Could you check a few things on this model? Use its own coordinates, in mm. A direction names the side the tool comes from. Coordinates: 2 decimals unless noted, no trailing zeros. Order: outer loops, then holes, each group sorted by start corner. A loop starts at its lowest first (then second) coordinate and runs counter-clockwise, first axis right, second up. Notation, with made-up numbers: (-5, 76) -> (10, 76) arc R13 ccw to (10, 88) -> close; hole circle Ø3 at (60, 3). An arc over 180 degrees is marked (long way). Use a Markdown table: item, result. Add a question column.
1) If we section it at C-C (x = -18): Write out the boundary of the cut face in (y, z).
2) Will these pins go through, and if not, where does the flat tip stop? pin 1 Ø0.8 at (y, z) = (5.5, 0.5) entering from +X; pin 2 Ø0.5 at (y, z) = (4.5, 0.5) entering from -X; pin 3 Ø0.5 at (x, z) = (-13.5, 1) entering from +Y; pin 4 Ø2.5 at (x, y) = (0, 18.415) entering from +Z.
3) If we section it at D-D (z = 0.9): Write out the boundary of the cut face in (x, y) (1 decimal), plus the area to 3 significant figures.
4) If we section it at A-A (x = 0): Write out the boundary of the cut face in (y, z), plus the area to 3 significant figures.
5) Which directions (+Z, -Z, +X, -X, +Y, -Y) give clear straight access to the entire face, cutting with the end or side of a thin tool? Please do faces 5 (the flat face through (-16.984, -4, 1)), 6 (the flat face through (0, -4, 0)), 7 (the flat face through (-2.007, -10.091, 0.783)).
6) Thinking about a two-plate mould opening in X: for faces 1 (the flat face through (-19, -5.524, 1)), 2 (the flat face through (-7.925, 5, 1)), 3 (the cylindrical face through (21.572, -0.871, 0.783)), 4 (the flat face through (-16.984, 4, 1)), which applies, +X half, -X half, draft (parallel to the pull), parting line (faces both ways), or undercut?
7) If I drill on L1, parallel to Y at x = 0, z = 1.05; L2, parallel to X at y = 6, z = 1.35; L3, parallel to X at y = 0, z = 1, over which ranges is the centre line in solid material (lowest first)? Write a range as [from, to].
8) If we section it at B-B (y = 0): Write out the boundary of the cut face in (x, z).
```python
from build123d import *

# Parameters (mm, degrees)
SKETCH1_R           = 1.4224
BOSS_EXTRUDE2_DEPTH = 1.5875


with BuildPart() as part:
    # Sketch1 → Boss-Extrude2 (new body)
    with BuildSketch(Plane.XY):
        with BuildLine():
            Line((-7.9248, 3.302), (-11.65986156, 2.948480848))
            Line((-11.65986156, 2.948480848), (-11.65986156, -2.948480848))
            Line((-11.65986156, -2.948480848), (-16.984058744, -2.948480848))
            Line((-16.984058744, -2.948480848), (-16.984058744, -5.5245))
            Line((-16.984058744, -5.5245), (-20.871224203, -5.5245))
            ThreePointArc((-20.871224203, -5.5245), (21.59, 0), (-20.871224203, 5.5245))
            Line((-20.871224203, 5.5245), (-16.984058744, 5.5245))
            Line((-16.984058744, 5.5245), (-16.984058744, 2.948480848))
            Line((-16.984058744, 2.948480848), (-14.952058744, 2.948480848))
            ThreePointArc((-14.952058744, 2.948480848), (-13.968818521, 6.093415226), (-12.332576282, 8.9535))
            Line((-12.332576282, 8.9535), (-7.9248, 7.366))
            Line((-7.9248, 7.366), (-7.9248, 3.302))
        make_face()
        with Locations((0, -18.415)):
            Circle(SKETCH1_R, mode=Mode.SUBTRACT)
        Polygon((-10.36446156, -3.837480848), (-8.512343898, -1.936173756), (-2.917588579, -7.386185056), (-2.594132624, -7.054138602), (-0.7747, -8.8265), (-3.273729572, -11.3919), (-5.093162196, -9.619538602), (-4.769706241, -9.287492148), align=None, mode=Mode.SUBTRACT)
        with Locations((0, 18.415)):
            Circle(SKETCH1_R, mode=Mode.SUBTRACT)
        with BuildLine():
            Line((11.43, 14.6558), (11.43, -0.8128))
            Line((11.43, -0.8128), (-5.6007, -0.8128))
            Line((-5.6007, -0.8128), (-5.6007, 14.173558463))
            ThreePointArc((-5.6007, 14.173558463), (-4.895856129, 14.43219293), (-4.179129857, 14.6558))
            Line((-4.179129857, 14.6558), (4.179129857, 14.6558))
            Line((4.179129857, 14.6558), (11.43, 14.6558))
        make_face(mode=Mode.SUBTRACT)
    extrude(amount=BOSS_EXTRUDE2_DEPTH)


solid = part.part
```
Answer sheet:
| question | item | result |
|---|---|---|
| 1 | outline | (-11.92, 0) -> (-5.52, 0) -> (-5.52, 1.59) -> (-11.92, 1.59) -> close; (5.52, 0) -> (11.92, 0) -> (11.92, 1.59) -> (5.52, 1.59) -> close |
| 2 | pin 1 | x = 20.98 |
| 2 | pin 2 | x = -16.98 |
| 2 | pin 3 | y = 17.05 |
| 2 | pin 4 | through |
| 3 | outline | (-20.9, -5.5) arc R21.6 ccw (long way) to (-20.9, 5.5) -> (-17, 5.5) -> (-17, 2.9) -> (-15, 2.9) arc R15.2 cw to (-12.3, 9) -> (-7.9, 7.4) -> (-7.9, 3.3) -> (-11.7, 2.9) -> (-11.7, -2.9) -> (-17, -2.9) -> (-17, -5.5) -> close; hole (-10.4, -3.8) -> (-4.8, -9.3) -> (-5.1, -9.6) -> (-3.3, -11.4) -> (-0.8, -8.8) -> (-2.6, -7.1) -> (-2.9, -7.4) -> (-8.5, -1.9) -> close; hole (-5.6, -0.8) -> (11.4, -0.8) -> (11.4, 14.7) -> (-4.2, 14.7) arc R15.2 ccw to (-5.6, 14.2) -> close; hole circle Ø2.8 at (0, -18.4); hole circle Ø2.8 at (0, 18.4) |
| 3 | area | 1,050 mm2 |
| 4 | outline | (-21.59, 0) -> (-19.84, 0) -> (-19.84, 1.59) -> (-21.59, 1.59) -> close; (-16.99, 0) -> (-0.81, 0) -> (-0.81, 1.59) -> (-16.99, 1.59) -> close; (14.66, 0) -> (16.99, 0) -> (16.99, 1.59) -> (14.66, 1.59) -> close; (19.84, 0) -> (21.59, 0) -> (21.59, 1.59) -> (19.84, 1.59) -> close |
| 4 | area | 35.0 mm2 |
| 5 | face 5 | +Z, -Z, -X |
| 5 | face 6 | -Z, +X, -X, +Y, -Y |
| 5 | face 7 | +Z, -Z |
| 6 | face 1 | draft |
| 6 | face 2 | undercut |
| 6 | face 3 | parting line |
| 6 | face 4 | -X half |
| 7 | L1 | [-21.59, -19.84], [-16.99, -0.81], [14.66, 16.99], [19.84, 21.59] |
| 7 | L2 | [-20.74, -14.01], [-7.92, -5.6], [11.43, 20.74] |
| 7 | L3 | [-11.66, -5.6], [11.43, 21.59] |
| 8 | outline | (-11.66, 0) -> (-5.6, 0) -> (-5.6, 1.59) -> (-11.66, 1.59) -> close; (11.43, 0) -> (21.59, 0) -> (21.59, 1.59) -> (11.43, 1.59) -> close |
